Part model, mm, in its own coordinate system. Face numbers are marked on the shaded views. A direction names the side the tool comes from. Round coordinates to 2 decimals unless told otherwise and drop trailing zeros. Loops run counter-clockwise (first coordinate to the right, second up) from the corner with the lowest first, then second, coordinate; pieces in that order, holes last.
from build123d import *

# Parameters (mm, degrees)
F0_W      = 110
F0_H      = 160
F0_W_2    = 22
F0_H_2    = 16
F1_DEPTH  = 3
F2_W      = 110
F2_H      = 160
F2_W_2    = 107
F2_H_2    = 157
F3_DEPTH  = 25.4
F5_D      = 16.4
F5_DEPTH  = 7.62
F6_D      = 4
F6_DEPTH  = 7.62
F7_D      = 12
F7_DEPTH  = 7.62
F8_SIZE   = 1
F9_SIZE   = 2.54
F10_R     = 10.1
F11_DEPTH = 12.7


with BuildPart() as f1:
    # F0 (on Top) → F1 (new body)
    with BuildSketch(Plane.XY):
        Rectangle(F0_W, F0_H)
        with Locations((0, -37.821583)):
            Rectangle(F0_W_2, F0_H_2, mode=Mode.SUBTRACT)
    extrude(amount=F1_DEPTH)

    # F2 (on face) → F3 (join)
    with BuildSketch(Plane(origin=(0, 0, 0), x_dir=(1, 0, 0), z_dir=(0, 0, -1))):
        Rectangle(F2_W, F2_H)
        Rectangle(F2_W_2, F2_H_2, mode=Mode.SUBTRACT)
    extrude(amount=F3_DEPTH)

    # F5
    with Locations(Plane.XZ.offset(80)):
        with Locations((29.456884, -11.2)):
            Hole(F5_D / 2, depth=F5_DEPTH)

    # F6
    with Locations(Plane.XZ.offset(80)):
        with Locations((0, -11.2)):
            Hole(F6_D / 2, depth=F6_DEPTH)

    # F7
    with Locations(Plane.XZ.offset(80)):
        with Locations((-30.313604, -11.2)):
            Hole(F7_D / 2, depth=F7_DEPTH)

    # F8
    f8_edges = [f1.edges().sort_by_distance(p)[0] for p in [
        (53.5, 0, -25.4),
        (0, 78.5, -25.4),
        (-53.5, 0, -25.4),
        (0, -78.5, -25.4),
    ]]
    chamfer(f8_edges, length=F8_SIZE)

    # F9
    f9_edges = [f1.edges().sort_by_distance(p)[0] for p in [
        (0, -45.821583, 3),
        (-11, -37.821583, 3),
        (11, -37.821583, 3),
        (-55, 0, 3),
        (0, -80, 3),
        (55, 0, 3),
        (0, 80, 3),
        (0, -29.821583, 3),
    ]]
    chamfer(f9_edges, length=F9_SIZE)

    # F10 (on face) → F11 (cut, symmetric)
    with BuildSketch(Plane(origin=(-55, 0, 0), x_dir=(0, -1, 0), z_dir=(-1, 0, 0))):
        with Locations((0, -12.47)):
            Circle(F10_R)
    extrude(amount=F11_DEPTH, both=True, mode=Mode.SUBTRACT)


solid = f1.part
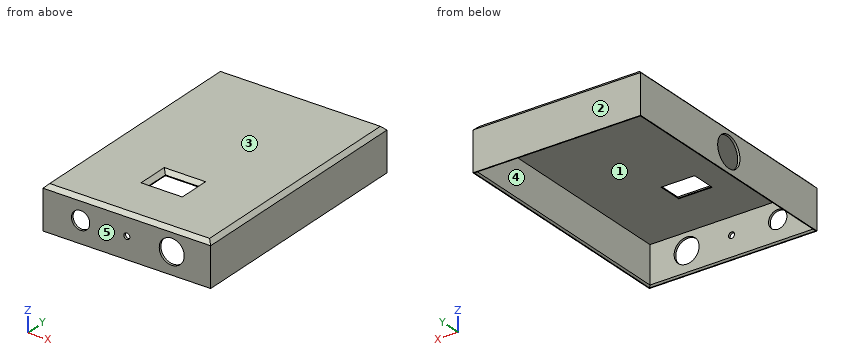
1) Slice it at B-B, the plane x = 0. Give the cut face in (y, z), then the cut area to 3 significant figures.
Values:
outline: (-80, -25.4) - (-79.5, -25.4) - (-78.5, -24.4) - (-78.5, -13.2) - (-80, -13.2) - close; (-80, -9.2) - (-78.5, -9.2) - (-78.5, 0) - (-45.82, 0) - (-45.82, 0.46) - (-48.36, 3) - (-77.46, 3) - (-80, 0.46) - close; (-29.82, 0) - (78.5, 0) - (78.5, -24.4) - (79.5, -25.4) - (80, -25.4) - (80, 0.46) - (77.46, 3) - (-27.28, 3) - (-29.82, 0.46) - close
area: 488 mm2
2) Mould opens along Y. For the marked faces 3, 4 and 5 say: released by +Y, released by -Y, zero draft, split by the parting line, or undercut.
Values:
face 3: zero draft
face 4: undercut
face 5: released by -Y
3) Slice it at D-D, the plane y = -53.5. Give the cut face in (x, z).
Values:
outline: (-55, -25.4) - (-54.5, -25.4) - (-53.5, -24.4) - (-53.5, 0) - (53.5, 0) - (53.5, -24.4) - (54.5, -25.4) - (55, -25.4) - (55, 0.46) - (52.46, 3) - (-52.46, 3) - (-55, 0.46) - close
4) Drop a flat-ended pin along its axis: pin 1 Ø1.5 at (x, y) = (13.5, 26.5) entering from -Z. Give the stop position or say it passes through.
Values:
pin 1: stops at z = 0
5) Slice it at A-A, the plane y = 0. Give the cut face in (x, z), then the cut area to 3 significant figures.
Values:
outline: (-55, -25.4) - (-54.5, -25.4) - (-53.5, -24.4) - (-53.5, -22.57) - (-55, -22.57) - close; (-55, -2.37) - (-53.5, -2.37) - (-53.5, 0) - (53.5, 0) - (53.5, -24.4) - (54.5, -25.4) - (55, -25.4) - (55, 0.46) - (52.46, 3) - (-52.46, 3) - (-55, 0.46) - close
area: 368 mm2
6) Tool access for the marked faces 1 and 2: list every direction of +Z, -Z, +X, -X, +Y, -Y with a clear straight run to the whole face (end or side of a thin tool).
Values:
face 1: -Z
face 2: +Z, -Z, +X, -X, +Y
7) Slice it at C-C, the plane x = 24. Give the cut face in (y, z).
Values:
outline: (-80, -25.4) - (-79.5, -25.4) - (-78.5, -24.4) - (-78.5, -17.32) - (-80, -17.32) - close; (-80, -5.08) - (-78.5, -5.08) - (-78.5, 0) - (78.5, 0) - (78.5, -24.4) - (79.5, -25.4) - (80, -25.4) - (80, 0.46) - (77.46, 3) - (-77.46, 3) - (-80, 0.46) - close
8) Wall check: line 1 along Y through (x, z) = (-37, -18.5); line 2 along X through (y, z) = (66, -23.25); line 3 along Y through (x, z) = (32, -9). Give the ranges that are in metal, low to high.
Values:
line 1: y = -80 to -78.5, 78.5 to 80
line 2: x = -55 to -53.5, 53.5 to 55
line 3: y = 78.5 to 80
